from build123d import *

# Parameters (mm, degrees)
F0_R     = 10.104738
F1_DEPTH = 25.4


with BuildPart() as f1:
    # F0 (on Top) → F1 (new body)
    with BuildSketch(Plane.XY):
        with BuildLine():
            ThreePointArc((36.215748, 1.502736), (19.263337, -8.635989), (15.140539, -27.953869))
            Line((15.140539, -27.953869), (0, -27.953869))
            Line((0, -27.953869), (0, -31.049898))
            Line((0, -31.049898), (11.078159, -31.049898))
            Line((11.078159, -31.049898), (11.161915, -31.049898))
            ThreePointArc((11.161915, -31.049898), (12.486345, -34.747137), (14.292773, -38.234328))
            Line((14.292773, -38.234328), (14.198601, -38.234328))
            Line((14.198601, -38.234328), (0, -38.234328))
            Line((0, -38.234328), (0, -42.281694))
            Line((0, -42.281694), (23.853084, -42.281694))
            ThreePointArc((23.853084, -42.281694), (58.692125, -38.479339), (54.755788, -3.655182))
            Line((54.755788, -3.655182), (54.755788, 56.323968))
            Line((54.755788, 56.323968), (36.215748, 56.323968))
            Line((36.215748, 56.323968), (36.215748, 1.502736))
        make_face()
        with BuildLine():
            ThreePointArc((50.319548, -7.202714), (38.556725, -42.249256), (29.828903, -6.326432))
            Line((29.828903, -6.326432), (31.886789, -9.716487))
            ThreePointArc((31.886789, -9.716487), (38.322899, -38.266224), (48.634886, -10.876921))
            Line((48.634886, -10.876921), (50.319548, -7.202714))
        make_face(mode=Mode.SUBTRACT)
        with BuildLine():
            Line((34.705213, -8.485508), (32.831621, -4.937194))
            ThreePointArc((32.831621, -4.937194), (40.139306, -3.803961), (47.334618, -5.510994))
            Line((47.334618, -5.510994), (45.750625, -9.145473))
            ThreePointArc((45.750625, -9.145473), (40.289779, -7.780181), (34.705213, -8.485508))
        make_face(mode=Mode.SUBTRACT)
        with BuildLine():
            Line((49.663853, 50.072402), (49.663853, 4.530995))
            ThreePointArc((49.663853, 4.530995), (45.465515, 5.751043), (41.132715, 6.335345))
            Line((41.132715, 6.335345), (41.132715, 50.072402))
            Line((41.132715, 50.072402), (49.663853, 50.072402))
        make_face(mode=Mode.SUBTRACT)
        with BuildLine():
            Line((0, -31.049898), (0, -27.953869))
            Line((0, -27.953869), (-34.656468, -27.953869))
            ThreePointArc((-34.656468, -27.953869), (-38.121079, -20.944111), (-44.953929, -17.142479))
            ThreePointArc((-44.953929, -17.142479), (-38.450523, -5.486514), (-44.018981, 6.643946))
            Line((-44.018981, 6.643946), (-44.018981, 18.070712))
            Line((-44.018981, 18.070712), (-49.515065, 9.375074))
            ThreePointArc((-49.515065, 9.375074), (-53.185694, 9.839214), (-56.856323, 9.375074))
            Line((-56.856323, 9.375074), (-62.085995, 17.700483))
            Line((-62.085995, 17.700483), (-62.085995, 6.850444))
            ThreePointArc((-62.085995, 6.850444), (-67.490664, -8.489032), (-55.495376, -19.471883))
            ThreePointArc((-55.495376, -19.471883), (-59.151883, -36.350704), (-42.931896, -42.281694))
            Line((-42.931896, -42.281694), (0, -42.281694))
            Line((0, -42.281694), (0, -38.234328))
            Line((0, -38.234328), (-37.386212, -38.234328))
            ThreePointArc((-37.386212, -38.234328), (-35.421086, -34.856351), (-34.536004, -31.049898))
            Line((-34.536004, -31.049898), (0, -31.049898))
        make_face()
        with Locations((-47.638755, -30.009355)):
            Circle(F0_R, mode=Mode.SUBTRACT)
        with BuildLine():
            ThreePointArc((-44.833815, 3.977288), (-52.410291, -17.076523), (-62.597681, 2.8454))
            Line((-62.597681, 2.8454), (-60.802351, 0.991043))
            ThreePointArc((-60.802351, 0.991043), (-52.559167, -14.52044), (-46.399061, 1.929766))
            Line((-46.399061, 1.929766), (-44.833815, 3.977288))
        make_face(mode=Mode.SUBTRACT)
        with BuildLine():
            Line((-59.396034, 2.457176), (-61.042475, 4.417974))
            ThreePointArc((-61.042475, 4.417974), (-53.702716, 7.275567), (-46.147241, 5.050103))
            Line((-46.147241, 5.050103), (-47.700324, 3.011949))
            ThreePointArc((-47.700324, 3.011949), (-53.642135, 4.715346), (-59.396034, 2.457176))
        make_face(mode=Mode.SUBTRACT)
        Polygon((-61.090183, 6.61603), (-61.090183, 13.13639), (-58.084256, 8.504227), align=None, mode=Mode.SUBTRACT)
        Polygon((-48.773948, 8.386992), (-45.554016, 13.13639), (-45.554016, 6.455034), align=None, mode=Mode.SUBTRACT)
    extrude(amount=F1_DEPTH)


solid = f1.part
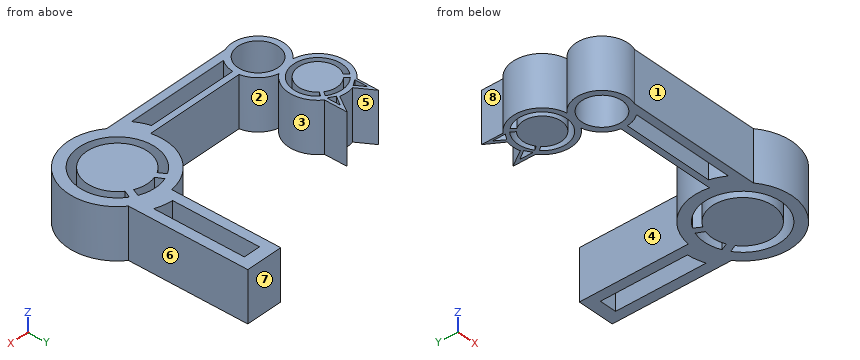
Part model, mm, in its own coordinate system. Face numbers are marked on the shaded views. A direction names the side the tool comes from. Give positions to 0.01 mm unless a question says otherwise; leave off trailing zeros. Order: outer loops, then holes, each group sorted by start corner. A loop starts at its lowest first (then second) coordinate and runs counter-clockwise, first axis right, second up. Notation, with made-up numbers: (-34.5, 62) - (14.5, 62) arc R37 cw to (14.5, 101) - close; hole circle Ø10 at (50.5, -15.75). An arc over 180 degrees is marked (long way). One line per question, with ' | ' between items.
1. Pull direction Y, two halves, no side cores. Call the marked faces 1, 2, 3 and 4: +Y half, -Y half, draft (parallel to the pull), parting line (faces both ways), or undercut.
Filled in:
face 1: -Y half | face 2: undercut | face 3: undercut | face 4: draft
2. Band-saw the part on B-B on x = -21. List the corners of the cut face in (y, z).
Filled in:
outline: (-42.28, 0) - (-38.23, 0) - (-38.23, 25.4) - (-42.28, 25.4) - close; (-31.05, 0) - (-27.95, 0) - (-27.95, 25.4) - (-31.05, 25.4) - close
3. Band-saw the part on D-D on z = 6.5. Give the number of separate pieces and of enclosed holes in the cut face, then the cut area to 3 significant figures.
Filled in:
separate pieces: 1 | enclosed holes: 9 | area: 3,380 mm²
4. Band-saw the part on A-A on y = 21.5. List the corners of the cut face in (x, z).
Filled in:
outline: (36.22, 0) - (41.13, 0) - (41.13, 25.4) - (36.22, 25.4) - close; (49.66, 0) - (54.76, 0) - (54.76, 25.4) - (49.66, 25.4) - close
5. Which spindle directions (+Z, -Z, +X, -X, +Y, -Y) get a long thin tool onto all of the face, cutting with end or side? Do the marked faces 5, 6, 7 and 8. Say none if no direction does.
Filled in:
face 5: +Z, -Z, +Y | face 6: +Z, -Z, +X, +Y | face 7: +Z, -Z, +X, -X, +Y | face 8: +Z, -Z, -X, +Y
6. Band-saw the part on C-C on y = -26. List the corners of the cut face in (x, z).
Filled in:
outline: (-60.16, 0) - (-56.91, 0) - (-56.91, 25.4) - (-60.16, 25.4) - close; (-38.36, 0) - (-35.12, 0) - (-35.12, 25.4) - (-38.36, 25.4) - close; (14.82, 0) - (20.37, 0) - (20.37, 25.4) - (14.82, 25.4) - close; (24.4, 0) - (54.36, 0) - (54.36, 25.4) - (24.4, 25.4) - close; (58.39, 0) - (63.93, 0) - (63.93, 25.4) - (58.39, 25.4) - close
7. Drill centre lines: probe 1 along Y at (x, z) = (39.5, 11); probe 2 along Y at (x, z) = (-4, 15.5); probe 3 along Y at (x, z) = (36, 22.75). Where is each one in solid material? Low to high.
Filled in:
probe 1: -47.76 to -42.27, -38.3 to -7.75, -3.79 to 56.32 | probe 2: -42.28 to -38.23, -31.05 to -27.95 | probe 3: -47.53 to -41.97, -37.92 to -8.13, -4.09 to 1.47
8. Drop flat-ended pins along their axis: P1, Ø12.5, axis at x = -10, z = 11, coming from the +Y side; P2, Ø12, axis at y = 15, z = 15.5, coming from the -X side; P3, Ø12.5, axis at x = -22.5, z = 12.5, coming from the -Y side. Give the stop position or say it passes through.
Filled in:
P1: y = -27.95 | P2: x = -62.09 | P3: y = -42.28
